Part model, mm, in its own coordinate system. Face numbers are marked on the shaded views. A direction names the side the tool comes from. Round coordinates to 2 decimals unless told otherwise and drop trailing zeros. Write each loop counter-clockwise with the first axis right and the second up, starting at its lowest first coordinate (ties: lowest second). Pieces come first, ordered by that corner, then holes. Notation, with made-up numbers: M 48,31.25 L 105,31.25 A28 cw 105,64.25 Z; hole C 10,83 d5. An arc over 180 degrees is marked long. Answer as a JSON object with one key per item and string values. Group by question number.
1. Drill centre lines: line 1 (Z direction, x = 120, y = 8.5); line 2 (X direction, y = 8.75, z = -2); line 3 (Z direction, x = 77.5, y = 3.5). Where is each one in solid material? Low to high. Write a range as from..to.
2. Band-saw the part on C-C, the plane y = 7.75. Write the cut outline in (x, z), plus the area to 3 significant figures.
3. Band-saw the part on D-D, the plane z = -17.5. Write the cut outline in (x, y), plus the area to 3 significant figures.
4. Two-plate mould, pull along X, no slides. Class the marked faces 1, 2, 3 and 4: +X half, -X half, draft (parallel to the pull), parting line (faces both ways), or undercut.
5. Which spindle directions (+Z, -Z, +X, -X, +Y, -Y) get a long thin tool onto all of the face, cutting with end or side? Do the marked faces 5, 6 and 7. Say none if no direction does.
6. Band-saw the part on A-A, the plane x = 0. Write the cut outline in (y, z), plus the area to 3 significant figures.
7. Band-saw the part on B-B, the plane z = 0. Write the cut outline in (x, y).
8. Drop flat-ended pins along their axis: pin 1 (8 mm diameter, centred on y = 9, z = 7.5, fed in from -X); pin 2 (5 mm diameter, centred on y = 5.5, z = 14, fed in from -X); pin 3 (1.5 mm diameter, centred on y = 11.5, z = -6, fed in from +X). Give the stop position or say it passes through.
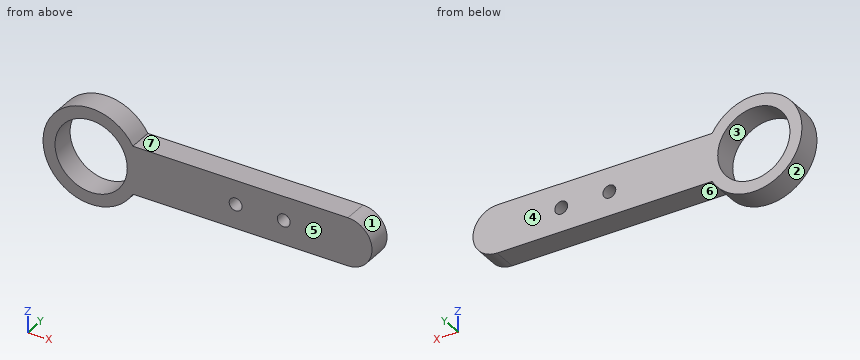
Autodesk Inventor part; units mm, degrees
ref_plane "YZ Plane" through (0, 0, 0) normal (1, 0, 0) x (0, 1, 0)
ref_plane "XZ Plane" through (0, 0, 0) normal (0, 1, 0) x (-1, 0, 0)
ref_plane "XY Plane" through (0, 0, 0) normal (0, 0, 1) x (1, 0, 0)
sketch "Sketch1" plane through (0, 0, 0) normal (0, 1, 0) x (-1, 0, 0)
  point P0 (0, 0)
sketch "Sketch2" plane through (0, 0, 0) normal (0, 1, 0) x (-1, 0, 0)
  arc A0 (-25.9808, -15) -> (-25.9808, 15) centre (0, 0) ccw
  line L0 (-160, 15) -> (-25.9808, 15)
  arc A1 (-160, 15) -> (-160, -15) centre (-160, 0) ccw
  line L1 (-25.9808, -15) -> (-160, -15)
  dimension "d1" = 60
  dimension "d4" = 30
extrude "Extrusion1" add sketch "Sketch2" along normal blind 15
sketch "Sketch3" plane through (0, 0, 0) normal (0, -1, 0) x (1, 0, 0)
  circle A0 centre (0, 0) radius 22.5
  circle A1 centre (90, 0) radius 4
  line L0 (0, 0) -> (120, 0)
  circle A2 centre (120, 0) radius 4
  dimension "d7" = 45
  dimension "d17" = 8
  dimension "d18" = 120
  dimension "d19" = 8
extrude "Extrusion2" cut sketch "Sketch3" against normal blind 15
Worked answers:
{
 "1": {"line 1": "z = -15..-4, 4..15", "line 2": "x = -29.93..-22.41, 22.41..86.54, 93.46..116.54, 123.46..174.87", "line 3": "z = -15..15"},
 "2": {"outline": "M 25.98,-15 L 160,-15 A15 ccw 160,15 L 25.98,15 A30 ccw long Z; hole C 0,0 d45; hole C 90,0 d8; hole C 120,0 d8", "area": "5,430 mm^2"},
 "3": {"outline": "M -24.37,0 L -14.14,0 L -14.14,15 L -24.37,15 Z; M 14.14,0 L 24.37,0 L 24.37,15 L 14.14,15 Z", "area": "307 mm^2"},
 "4": {"face 1": "+X half", "face 2": "parting line", "face 3": "undercut", "face 4": "draft"},
 "5": {"face 5": "+Z, -Z, +X, -X, -Y", "face 6": "-Z, +X, +Y, -Y", "face 7": "+Z, +X, +Y, -Y"},
 "6": {"outline": "M 0,-30 L 15,-30 L 15,-22.5 L 0,-22.5 Z; M 0,22.5 L 15,22.5 L 15,30 L 0,30 Z", "area": "225 mm^2"},
 "7": {"outline": "M -30,0 L -22.5,0 L -22.5,15 L -30,15 Z; M 22.5,0 L 86,0 L 86,15 L 22.5,15 Z; M 94,0 L 116,0 L 116,15 L 94,15 Z; M 124,0 L 175,0 L 175,15 L 124,15 Z"},
 "8": {"pin 1": "stops at x = -29.8", "pin 2": "stops at x = -27.71", "pin 3": "stops at x = 174.05"}
}
